Verification items for the finished model (mm, model axes). A direction names the side the tool comes from. Round coordinates to 2 decimals unless told otherwise and drop trailing zeros. Write each loop counter-clockwise with the first axis right and the second up, starting at its lowest first coordinate (ties: lowest second). Pieces come first, ordered by that corner, then holes. Notation, with made-up numbers: (26, 36) - (52, 36) arc R17 ccw to (52, 48) - close; hole circle Ø11 at (31.5, -25.5). An arc over 180 degrees is marked (long way). Answer as a JSON object with one key per item and string values.
```python
from build123d import *

# Parameters (mm, degrees)
SALIENTE_EXTRUIR2_DEPTH = 50
CROQUIS4_R              = 1.5
CORTAR_EXTRUIR2_DEPTH   = 95


with BuildPart() as part:
    # Croquis2 → Saliente-Extruir2 (new body)
    with BuildSketch(Plane(origin=(0, 0, 0), x_dir=(0, 0, -1), z_dir=(1, 0, 0))):
        Polygon((-34.418181818, 2.5), (-34.418181818, 22.5), (-29.418181818, 22.5), (-29.418181818, 2.5), (-25.218181818, 2.5), (-25.218181818, 22.5), (-20.218181818, 22.5), (-20.218181818, 2.5), (27.281818182, 2.5), (27.281818182, 22.5), (32.281818182, 22.5), (32.281818182, 2.5), (36.481818182, 2.5), (36.481818182, 22.5), (41.481818182, 22.5), (41.481818182, 2.5), (41.481818182, -2.5), (-34.418181818, -2.5), align=None)
    extrude(amount=SALIENTE_EXTRUIR2_DEPTH)

    # Croquis4 → Cortar-Extruir2 (cut)
    with BuildSketch(Plane.XY.offset(34.418181818)):
        with Locations(Location((15, 12.5, 0), (0, 0, 270))):
            Circle(CROQUIS4_R)
        with Locations(Location((35, 12.5, 0), (0, 0, 270))):
            Circle(CROQUIS4_R)
    extrude(amount=-CORTAR_EXTRUIR2_DEPTH, mode=Mode.SUBTRACT)


solid = part.part
```
1. Cross-section at C-C (x = 46). Record the boundary of the cut face in (y, z).
Completed:
{"outline": "(-2.5, -41.48) - (22.5, -41.48) - (22.5, -36.48) - (2.5, -36.48) - (2.5, -32.28) - (22.5, -32.28) - (22.5, -27.28) - (2.5, -27.28) - (2.5, 20.22) - (22.5, 20.22) - (22.5, 25.22) - (2.5, 25.22) - (2.5, 29.42) - (22.5, 29.42) - (22.5, 34.42) - (-2.5, 34.42) - close"}
2. Cross-section at B-B (x = 35). Count the separate pieces of the cut face and the enclosed holes in it, plus the area to 4 significant figures.
Completed:
{"separate pieces": "5", "enclosed holes": "0", "area": "719.5 mm^2"}
3. Mould release check, pull along Y, two halves, no side actions. Record for faces 1 (the face through (25, 2.5, -3)), 2 (the face through (25, 13, 29.418)), 3 (the face through (16.01, 13.61, -29.75)): released by +Y, released by -Y, zero draft, split by the parting line, or undercut.
Completed:
{"face 1": "released by +Y", "face 2": "zero draft", "face 3": "undercut"}
4. Cross-section at A-A (y = 9.25). Record the boundary of the cut face in (x, z), plus the area to 3 significant figures.
Completed:
{"outline": "(0, -41.48) - (50, -41.48) - (50, -36.48) - (0, -36.48) - close; (0, -32.28) - (50, -32.28) - (50, -27.28) - (0, -27.28) - close; (0, 20.22) - (50, 20.22) - (50, 25.22) - (0, 25.22) - close; (0, 29.42) - (50, 29.42) - (50, 34.42) - (0, 34.42) - close", "area": "1,000 mm^2"}
5. Access from +Z, -Z, +X, -X, +Y, -Y to the whole of each face (thin tool, end or side, straight path). Record for faces 4 (the face through (25, 2.5, 27)), 5 (the face through (33.536, 12.825, -29.747)).
Completed:
{"face 4": "+X, -X, +Y", "face 5": "+Z, -Z"}
6. Material ranges on probe 1 along X at (y, z) = (12.5, 30.65); probe 2 along Z at (x, y) = (45.5, 20.25); probe 3 along Y at (x, z) = (7, -36), recorded low to high. Write a range as from..to.
Completed:
{"probe 1": "x = 0..13.5, 16.5..33.5, 36.5..50", "probe 2": "z = -41.48..-36.48, -32.28..-27.28, 20.22..25.22, 29.42..34.42", "probe 3": "y = -2.5..2.5"}
7. Cross-section at D-D (z = -9). Record the boundary of the cut face in (x, y), plus the area to 3 significant figures.
Completed:
{"outline": "(0, -2.5) - (50, -2.5) - (50, 2.5) - (0, 2.5) - close", "area": "250 mm^2"}
8. Go/stop test with flat-tipped pins: pin 1 (10 mm diameter, centred on x = 36, y = 13, fed in from +Z); pin 2 (1.8 mm diameter, centred on x = 15, y = 12.5, fed in from -Z); pin 3 (14 mm diameter, centred on x = 24, z = -5, fed in from +Y). Record where each tip stops, or that it passes through.
Completed:
{"pin 1": "stops at z = 34.42", "pin 2": "passes through", "pin 3": "stops at y = 2.5"}
